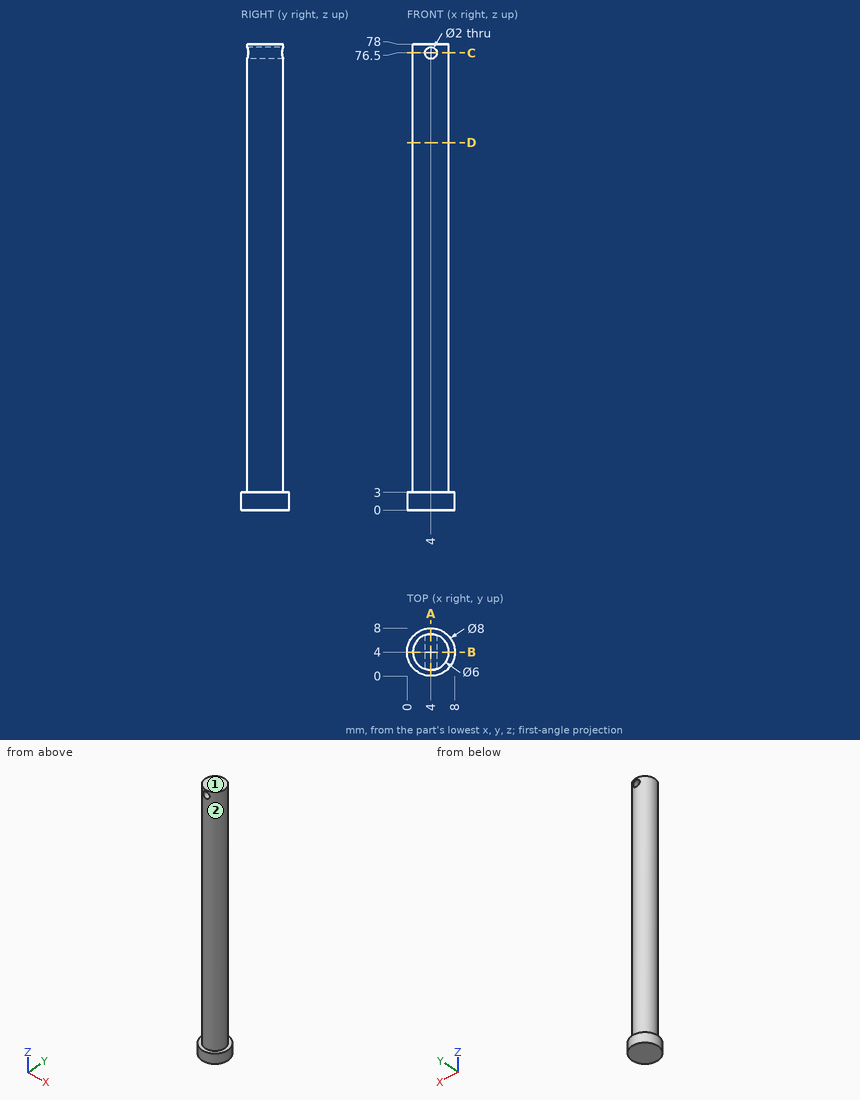
Can you work these out from the drawing? Everything is in mm from the part's minimum corner. A direction names the side the tool comes from. Round coordinates to 2 decimals unless told otherwise and drop trailing zeros. Loops run counter-clockwise (first coordinate to the right, second up) from the corner with the lowest first, then second, coordinate; pieces in that order, holes last. Notation, with made-up numbers: M 84,-36.75 L 116,-36.75 A11 cw 116,-18.75 Z; hole C -16.5,6 d11. An arc over 180 degrees is marked long. Answer in a Markdown table with one row per item.
1. If we section it at D-D, the plane z = 61.5: Please give me the cut outline in (x, y).
Established:
| item | result |
|---|---|
| outline | C 4,4 d6 |
2. On a 3-axis mill with a long thin cutter (end or side, diameter ignored), from which of +Z, -Z, +X, -X, +Y, -Y can I reach the whole of each face in a straight line? I mean the marked faces 1 and 2. Say none if no direction works.
Established:
| item | result |
|---|---|
| face 1 | +Z, +X, -X, +Y, -Y |
| face 2 | +Z |
3. If we section it at B-B, the plane y = 4: Please give me the cut outline in (x, z).
Established:
| item | result |
|---|---|
| outline | M 0,0 L 8,0 L 8,3 L 7,3 L 7,78 L 1,78 L 1,3 L 0,3 Z; hole C 4,76.5 d2 |
4. Please list where these lines run through material, in increasing order: line 1 (Z direction, x = 4, y = 4.5); line 2 (Z direction, x = 0.5, y = 3); line 3 (Z direction, x = 4.75, y = 3.5). Write a range as from..to.
Established:
| item | result |
|---|---|
| line 1 | 0..75.5, 77.5..78 |
| line 2 | 0..3 |
| line 3 | 0..75.84, 77.16..78 |
5. I'm going to push flat-ended pins straight in: pin 1 Ø1 at (x, z) = (4.5, 16.5) entering from -Y; pin 2 Ø2 at (y, z) = (5.5, 29.5) entering from -X; pin 3 Ø2.5 at (x, z) = (4, 76.5) entering from +Y. Where does each tip first touch, or does it pass through?
Established:
| item | result |
|---|---|
| pin 1 | y = 1 |
| pin 2 | x = 1.04 |
| pin 3 | y = 7 |
6. If we section it at C-C, the plane z = 76.5: Please give me the cut outline in (x, y), plus the area to 3 significant figures.
Established:
| item | result |
|---|---|
| outline | M 3,1.17 L 3,6.83 A3 ccw Z; M 5,1.17 A3 ccw 5,6.83 Z |
| area | 16.5 mm² |
7. If we section it at A-A, the plane x = 4: Please give me the cut outline in (y, z).
Established:
| item | result |
|---|---|
| outline | M 0,0 L 8,0 L 8,3 L 7,3 L 7,75.5 L 1,75.5 L 1,3 L 0,3 Z; M 1,77.5 L 7,77.5 L 7,78 L 1,78 Z |
